Read the model definition and answer for the solid it produces. Units are mm, in the model's axes. Face numbers are marked on the shaded views. A direction names the side the tool comes from. Give positions to 0.01 mm unless a question says otherwise; leave off trailing zeros. Return JSON: item names as keys, results as strings.
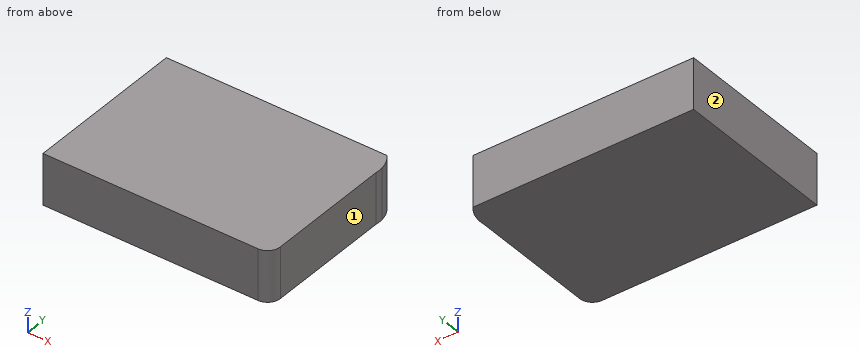
```python
from build123d import *

# Parameters (mm, degrees)
F1_DEPTH = 25.4


with BuildPart() as f1:
    # F0 (on Top) → F1 (new body)
    with BuildSketch(Plane.XY):
        with BuildLine():
            Line((25.366824, 43.394551), (-61.614241, 43.394551))
            Line((-61.614241, 43.394551), (-61.614241, -37.99203))
            Line((-61.614241, -37.99203), (45.545957, -37.99203))
            ThreePointArc((45.545957, -37.99203), (50.036086, -36.132158), (51.895957, -31.64203))
            Line((51.895957, -31.64203), (51.895957, 31.554978))
            ThreePointArc((51.895957, 31.554978), (30.702339, 19.708002), (25.366824, 43.394551))
        make_face()
        with BuildLine():
            Line((48.386586, 43.394551), (25.366824, 43.394551))
            ThreePointArc((25.366824, 43.394551), (30.702339, 19.708002), (51.895957, 31.554978))
            Line((51.895957, 31.554978), (51.895957, 35.531041))
            ThreePointArc((51.895957, 35.531041), (50.711712, 39.717375), (48.386586, 43.394551))
        make_face()
        with BuildLine():
            Line((51.895957, 35.531041), (51.895957, 31.554978))
            ThreePointArc((51.895957, 31.554978), (52.02696, 33.543009), (51.895957, 35.531041))
        make_face()
    extrude(amount=F1_DEPTH)


solid = f1.part
```
Q1. For the marked faces 1 and 2, determine the directions among +Z, -Z, +X, -X, +Y, -Y from which every point of the face is accessible in a straight line to the end or side of a thin tool.
Values:
{"face 1": "+Z, -Z, +X, -Y", "face 2": "+Z, -Z, -X, +Y, -Y"}
Q2. Given pin 1 (8 mm diameter, centred on x = 10, y = 15, fed in from -Z); pin 2 (3 mm diameter, centred on y = -22, z = 19.5, fed in from +X), each flat-ended and moving along its own axis, determine where each tip first touches the part or whether it passes through.
Values:
{"pin 1": "stops at z = 0", "pin 2": "stops at x = 51.9"}
Q3. Consider L1, parallel to X at y = 29, z = 23; L2, parallel to X at y = 36.5, z = 13. Determine where each line is inside the solid, lowest interval first.
Values:
{"L1": "x = -61.61 to 51.9", "L2": "x = -61.61 to 51.74"}
